For this review, take the finished solid that the model builds, in its own axes (mm). Coordinates: 2 decimals unless noted, no trailing zeros. Write each loop counter-clockwise with the first axis right and the second up, starting at its lowest first coordinate (ties: lowest second). Pieces come first, ordered by that corner, then holes. Notation, with made-up numbers: (12.25, 46.25) -> (25.25, 46.25) arc R32 ccw to (25.25, 80.25) -> close; hole circle Ø6 at (32, 69.5). An arc over 180 degrees is marked (long way). One line per item, written item: value. Start each with the question number.
1) Add section D-D (y = -96.5). State the section outline as (x, z) points, and give its area (3 significant figures).
2) Add section B-B (z = -49). State the section outline as (x, y) points.
3) For probe 1 along Z at (x, y) = (5, 3); probe 2 along Y at (x, z) = (5, -20); probe 3 along Y at (x, z) = (2, -50), list the stretches that pass through material, from the lowest coordinate up. Write a range as from..to.
4) Add section C-C (x = 4.75). State how many separate pieces and enclosed holes the cut face has, and give its area (3 significant figures).
5) For pin 1 Ø1.9 at (x, z) = (1.5, -25.5) entering from -Y; pin 2 Ø1.9 at (x, z) = (2.5, -68.5) entering from -Y; pin 3 Ø5 at (y, z) = (36, -23) entering from -X; pin 4 Ø1.9 at (x, z) = (2, -26.5) entering from +Y, all flat-tipped, find the tip position at first contact; note any pin that passes through.
6) Add section A-A (y = 71). State the section outline as (x, z) points, and give its area (3 significant figures).
from build123d import *

# Parameters (mm, degrees)
F0_W      = 220
F0_H      = 180
F1_DEPTH  = 6.2
F2_W      = 12
F2_H      = 6.2
F3_DEPTH  = 6.201
F5_DEPTH  = 6.201
F6_W      = 6.2
F6_H      = 12
F7_DEPTH  = 6.2
F8_W      = 6
F8_H      = 6.2
F8_W_2    = 12
F9_DEPTH  = 6.2
F10_W     = 2.2
F10_H     = 6.2
F11_DEPTH = 6.2


with BuildPart() as f1:
    # F0 (on Right) → F1 (new body)
    with BuildSketch(Plane.YZ):
        Rectangle(F0_W, F0_H)
    extrude(amount=F1_DEPTH)

    # F2 (on face) → F3 (cut, through all)
    with BuildSketch(Plane.YZ.offset(6.2)):
        with Locations((-96, -25.4)):
            Rectangle(F2_W, F2_H)
        with Locations((-72, -25.4)):
            Rectangle(F2_W, F2_H)
        with Locations((-48, -25.4)):
            Rectangle(F2_W, F2_H)
        with Locations((-24, -25.4)):
            Rectangle(F2_W, F2_H)
        with Locations((0, -25.4)):
            Rectangle(F2_W, F2_H)
        with Locations((24, -25.4)):
            Rectangle(F2_W, F2_H)
        with Locations((48, -25.4)):
            Rectangle(F2_W, F2_H)
        with Locations((72, -25.4)):
            Rectangle(F2_W, F2_H)
        with Locations((96, -25.4)):
            Rectangle(F2_W, F2_H)
    extrude(amount=-F3_DEPTH, mode=Mode.SUBTRACT)

    # F4 (on face) → F5 (cut, through all)
    with BuildSketch(Plane.YZ.offset(6.2)):
        Polygon((-84, -90), (-84, -28.5), (-90, -28.5), (-102, -28.5), (-110, -28.5), (-110, -90), align=None)
    extrude(amount=-F5_DEPTH, mode=Mode.SUBTRACT)

    # F6 (on face) → F7 (join)
    with BuildSketch(Plane.YZ.offset(6.2)):
        with Locations((113.1, 12)):
            Rectangle(F6_W, F6_H)
        with Locations((113.1, 36)):
            Rectangle(F6_W, F6_H)
        with Locations((113.1, 60)):
            Rectangle(F6_W, F6_H)
        with Locations((113.1, 84)):
            Rectangle(F6_W, F6_H)
        with Locations((113.1, -12)):
            Rectangle(F6_W, F6_H)
        with Locations((113.1, -36)):
            Rectangle(F6_W, F6_H)
        with Locations((113.1, -60)):
            Rectangle(F6_W, F6_H)
        with Locations((113.1, -84)):
            Rectangle(F6_W, F6_H)
        with Locations((-113.1, 12)):
            Rectangle(F6_W, F6_H)
        with Locations((-113.1, -12)):
            Rectangle(F6_W, F6_H)
        with Locations((-113.1, 36)):
            Rectangle(F6_W, F6_H)
        with Locations((-113.1, 84)):
            Rectangle(F6_W, F6_H)
        with Locations((-113.1, 60)):
            Rectangle(F6_W, F6_H)
    extrude(amount=-F7_DEPTH)

    # F8 (on face) → F9 (join)
    with BuildSketch(Plane.YZ.offset(6.2)):
        with Locations((-81, -93.1)):
            Rectangle(F8_W, F8_H)
        with Locations((-60, -93.1)):
            Rectangle(F8_W_2, F8_H)
        with Locations((-36, -93.1)):
            Rectangle(F8_W_2, F8_H)
        with Locations((-12, -93.1)):
            Rectangle(F8_W_2, F8_H)
        with Locations((12, -93.1)):
            Rectangle(F8_W_2, F8_H)
        with Locations((36, -93.1)):
            Rectangle(F8_W_2, F8_H)
        with Locations((60, -93.1)):
            Rectangle(F8_W_2, F8_H)
        with Locations((84, -93.1)):
            Rectangle(F8_W_2, F8_H)
        with Locations((108, -93.1)):
            Rectangle(F8_W_2, F8_H)
    extrude(amount=-F9_DEPTH)

    # F10 (on face) → F11 (join)
    with BuildSketch(Plane.YZ.offset(6.2)):
        with Locations((115.1, -93.1)):
            Rectangle(F10_W, F10_H)
    extrude(amount=-F11_DEPTH)


solid = f1.part
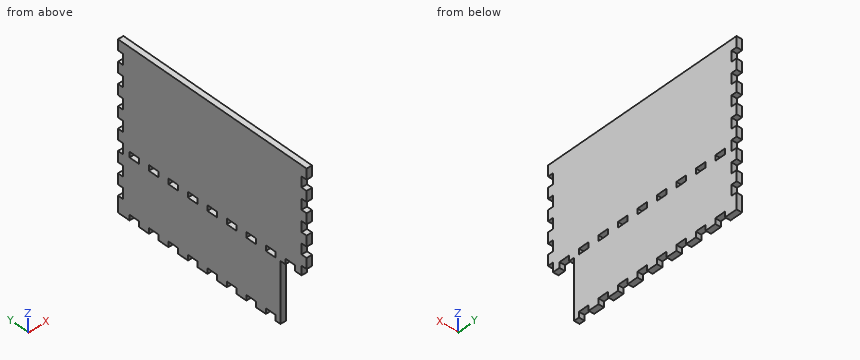
Numbers:
1. outline: (0, -22.3) -> (6.2, -22.3) -> (6.2, 90) -> (0, 90) -> close
1. area: 696 mm²
2. outline: (0, -84) -> (6.2, -84) -> (6.2, 110) -> (0, 110) -> close
3. probe 1: -90..-28.5, -22.3..90
3. probe 2: -110..110
3. probe 3: -84..110
4. separate pieces: 1
4. enclosed holes: 8
4. area: 38,900 mm²
5. pin 1: y = -110
5. pin 2: y = -84
5. pin 3: x = 0
5. pin 4: y = 110
6. outline: (0, -90) -> (6.2, -90) -> (6.2, -28.5) -> (0, -28.5) -> close; (0, -22.3) -> (6.2, -22.3) -> (6.2, 90) -> (0, 90) -> close
6. area: 1,080 mm²
